```python
from build123d import *

# Parameters (mm, degrees)
SKETCH_1_R          = 210
SKETCH_1_R_2        = 203
EXTRUDE_2_DEPTH     = 174
EXTRUDE_START       = -174
EXTRUDE_4_DEPTH     = 174
CUT_EXTRUDE_1_DEPTH = 654
EXTRUDE_5_DEPTH     = 174
EXTRUDE_6_DEPTH     = 174
EXTRUDE_7_DEPTH     = 174
EXTRUDE_8_DEPTH     = 174
EXTRUDE_9_DEPTH     = 174
SKETCH_11_R         = 55
CUT_EXTRUDE_4_DEPTH = 221.5
CUT_EXTRUDE_5_DEPTH = 87
SKETCH_13_W         = 252.379443355
SKETCH_13_H         = 197.496269512
CUT_EXTRUDE_6_DEPTH = 244


with BuildPart() as part:
    # 草图1 → 凸台-拉伸2 (new body)
    with BuildSketch(Plane.XY):
        Circle(SKETCH_1_R)
        Circle(SKETCH_1_R_2, mode=Mode.SUBTRACT)
    extrude(amount=EXTRUDE_2_DEPTH)

    # 草图2 → 凸台-拉伸4 (add)
    with BuildSketch(Plane.XY.offset(174).offset(EXTRUDE_START)):
        with BuildLine():
            Line((-170.735431044, -102), (-173.735431044, -102))
            Line((-173.735431044, -102), (-175.513532242, -102))
            ThreePointArc((-175.513532242, -102), (-174.63092392, -103.50381834), (-173.735431044, -105))
            Line((-173.735431044, -105), (-170.735431044, -105))
            Line((-170.735431044, -105), (-170.735431044, -102))
        make_face()
        with BuildLine():
            ThreePointArc((173.735431044, -105), (174.63092392, -103.50381834), (175.513532242, -102))
            Line((175.513532242, -102), (173.735431044, -102))
            Line((173.735431044, -102), (170.735431044, -102))
            Line((170.735431044, -102), (170.735431044, -105))
            Line((170.735431044, -105), (173.735431044, -105))
        make_face()
    extrude(amount=EXTRUDE_4_DEPTH)

    # 草图3 → 切除-拉伸1 (cut)
    with BuildSketch(Plane.XY.offset(174)):
        Polygon((-170.735431044, -102), (238.333646515, -102), (254.334169784, 272.292523591), (-334.569415043, 221.85110305), (-306.830562533, -102), align=None)
    extrude(amount=-CUT_EXTRUDE_1_DEPTH, mode=Mode.SUBTRACT)

    # 草图5 → 凸台-拉伸5 (add)
    with BuildSketch(Plane.XY.offset(174).offset(EXTRUDE_START)):
        with BuildLine():
            Line((-120, -209.75), (-10.243900624, -209.75))
            ThreePointArc((-10.243900624, -209.75), (-67.755470707, -198.769203322), (-120, -172.336879396))
            Line((-120, -172.336879396), (-120, -209.75))
        make_face()
        with BuildLine():
            ThreePointArc((120, -172.336879396), (67.755470707, -198.769203322), (10.243900624, -209.75))
            Line((10.243900624, -209.75), (120, -209.75))
            Line((120, -209.75), (120, -172.336879396))
        make_face()
    extrude(amount=EXTRUDE_5_DEPTH)

    # 草图6 → 凸台-拉伸6 (add)
    with BuildSketch(Plane.XY.offset(174).offset(EXTRUDE_START)):
        with BuildLine():
            Line((-175.513532242, -102), (-166.195667814, -102))
            ThreePointArc((-166.195667814, -102), (0, -195), (166.195667814, -102))
            Line((166.195667814, -102), (175.513532242, -102))
            ThreePointArc((175.513532242, -102), (0, -203), (-175.513532242, -102))
        make_face()
    extrude(amount=EXTRUDE_6_DEPTH)

    # 草图7 → 凸台-拉伸7 (add)
    with BuildSketch(Plane.XY.offset(174).offset(EXTRUDE_START)):
        with BuildLine():
            Line((-166.933126535, -92), (-166.933126535, -95))
            Line((-166.933126535, -95), (-170.293863659, -95))
            ThreePointArc((-170.293863659, -95), (0, -195), (170.293863659, -95))
            Line((170.293863659, -95), (166.933126535, -95))
            Line((166.933126535, -95), (166.933126535, -92))
            Line((166.933126535, -92), (171.933126535, -92))
            Line((171.933126535, -92), (188.496850106, -92))
            ThreePointArc((188.496850106, -92), (0, -209.75), (-188.496850106, -92))
            Line((-188.496850106, -92), (-171.933126535, -92))
            Line((-171.933126535, -92), (-166.933126535, -92))
        make_face()
    extrude(amount=EXTRUDE_7_DEPTH)

    # 草图8 → 凸台-拉伸8 (add)
    with BuildSketch(Plane(origin=(0, 0, 0), x_dir=(-1, 0, 0), z_dir=(0, 0, -1))):
        with BuildLine():
            Line((166.933126535, -92), (163.933126535, -92))
            Line((163.933126535, -92), (163.933126535, -99))
            Line((163.933126535, -99), (168, -99))
            ThreePointArc((168, -99), (169.158755456, -97.006780447), (170.293863659, -95))
            Line((170.293863659, -95), (166.933126535, -95))
            Line((166.933126535, -95), (166.933126535, -92))
        make_face()
        with BuildLine():
            Line((-166.933126535, -95), (-170.293863659, -95))
            ThreePointArc((-170.293863659, -95), (-169.158755456, -97.006780447), (-168, -99))
            Line((-168, -99), (-163.933126535, -99))
            Line((-163.933126535, -99), (-163.933126535, -92))
            Line((-163.933126535, -92), (-166.933126535, -92))
            Line((-166.933126535, -92), (-166.933126535, -95))
        make_face()
    extrude(amount=-EXTRUDE_8_DEPTH)

    # 草图9 → 凸台-拉伸9 (add)
    with BuildSketch(Plane.XY.offset(174).offset(EXTRUDE_START)):
        with BuildLine():
            ThreePointArc((10.243900624, -209.75), (5.123475383, -209.937490697), (0, -210))
            Line((0, -210), (0, -225))
            Line((0, -225), (18.007375678, -225))
            Line((18.007375678, -225), (120, -225))
            Line((120, -225), (120, -209.75))
            Line((120, -209.75), (10.243900624, -209.75))
        make_face()
        with BuildLine():
            Line((0, -225), (0, -210))
            ThreePointArc((0, -210), (-5.123475383, -209.937490697), (-10.243900624, -209.75))
            Line((-10.243900624, -209.75), (-120, -209.75))
            Line((-120, -209.75), (-120, -225))
            Line((-120, -225), (0, -225))
        make_face()
    extrude(amount=EXTRUDE_9_DEPTH)

    # 草图11 → 切除-拉伸4 (cut)
    with BuildSketch(Plane(origin=(0, 0, 0), x_dir=(1, 0, 0), z_dir=(0, 1, 0))):
        with Locations(Location((0, -87, 0), (0, 0, 270))):
            Circle(SKETCH_11_R)
    extrude(amount=-CUT_EXTRUDE_4_DEPTH, mode=Mode.SUBTRACT)

    # 草图10 → 切除-拉伸5 (cut)
    with BuildSketch(Plane.XY.offset(174)):
        Polygon((5, -221.5), (-5, -221.5), (-5, -211.5), (0, -211.5), (5, -211.5), align=None)
    extrude(amount=-CUT_EXTRUDE_5_DEPTH, mode=Mode.SUBTRACT)

    # 草图13 → 切除-拉伸6 (cut)
    with BuildSketch(Plane(origin=(0, 0, 0), x_dir=(0, 0, -1), z_dir=(1, 0, 0))):
        with Locations((-79.30804003, -159.33156324)):
            Rectangle(SKETCH_13_W, SKETCH_13_H)
    extrude(amount=-CUT_EXTRUDE_6_DEPTH, mode=Mode.SUBTRACT)


solid = part.part
```
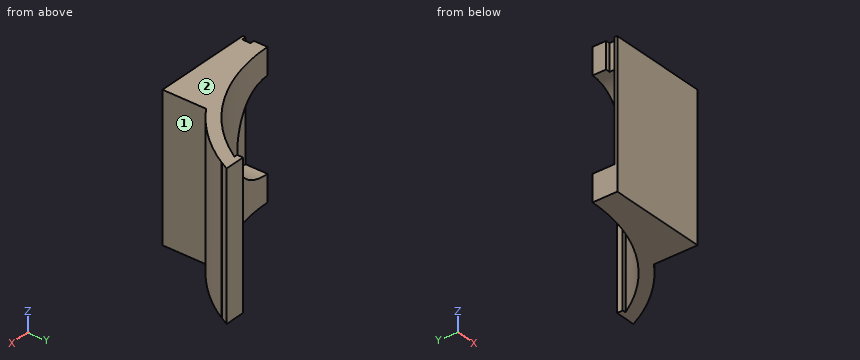
Input: part model. Units: mm. Frame: model coordinates. Face numbers are marked on the shaded views. A direction names the side the tool comes from. Coordinates: 2 decimals unless noted, no trailing zeros. Order: outer loops, then holes, each group sorted by start corner. A loop starts at its lowest first (then second) coordinate and runs counter-clockwise, first axis right, second up. Notation, with made-up numbers: (50.5, -36.5) - (76.5, -36.5) arc R28 ccw to (76.5, -5.5) - close; hole circle Ø2 at (44, 12). An arc over 180 degrees is marked (long way). Return JSON: item names as keys, results as strings.
Q1. Cut plane B-B (y = -206). Return loops of the section in (x, z).
The answers:
{"outline": "(0, 0) - (120, 0) - (120, 174) - (0, 174) - (0, 142) arc R55 cw to (0, 32) - close"}
Q2. First-contact query: pin 1 (4 mm diameter, centred on y = -137, z = 92, fed in from -X); pin 2 (4.5 mm diameter, centred on x = 165, z = 51.5, fed in from -Y); pin 3 (10 mm diameter, centred on y = -211.5, z = 78, fed in from +X). Flat tips, straight axial feed; report the tip coordinate or a pass-through.
The answers:
{"pin 1": "stops at x = 136.76", "pin 2": "stops at y = -132.71", "pin 3": "stops at x = 120"}
Q3. Access query for the marked faces 1 and 2. Directions: +Z, -Z, +X, -X, +Y, -Y. A direction counts if a zero-diameter tool reaches every point of the face in a straight line with its end or side. Return the directions, or none.
The answers:
{"face 1": "+Z, -Z, +X, -Y", "face 2": "+Z, +X, -X, +Y, -Y"}
Q4. Cut plane A-A (z = 87). Return loops of the section in (x, y).
The answers:
{"outline": "(0, -225) - (120, -225) - (120, -172.34) arc R210 ccw to (183.56, -102) - (183.28, -102) arc R209.75 ccw to (188.5, -92) - (163.93, -92) - (163.93, -99) - (168, -99) arc R195 cw to (55, -187.08) - (55, -221.5) - (0, -221.5) - close"}
Q5. Cut plane C-C (z = 162.5). Return loops of the section in (x, y), then the cut area to 3 significant figures.
The answers:
{"outline": "(0, -225) - (120, -225) - (120, -172.34) arc R210 ccw to (183.56, -102) - (183.28, -102) arc R209.75 ccw to (188.5, -92) - (163.93, -92) - (163.93, -99) - (168, -99) arc R195 cw to (0, -195) - (0, -211.5) - (5, -211.5) - (5, -221.5) - (0, -221.5) - close", "area": "6,580 mm2"}
Q6. Cut plane D-D (x = 68.5). Return loops of the section in (y, z), then the cut area to 3 significant figures.
The answers:
{"outline": "(-225, 0) - (-182.57, 0) - (-182.57, 174) - (-225, 174) - close", "area": "7,380 mm2"}
Q7. Ray query, probe 1 along X at (y, z) = (-105.5, 115.5); probe 2 along X at (y, z) = (-117, 154); probe 3 along Y at (x, z) = (104, 42.5). Return the intervals inside material, ascending.
The answers:
{"probe 1": "x = 164 to 181.58", "probe 2": "x = 156 to 174.39", "probe 3": "y = -225 to -164.95"}
